from build123d import *

# Parameters (mm, degrees)
SKETCH_1_R               = 7.5
EXTRUDE_1_DEPTH          = 5
SKETCH_2_R               = 7.5
SKETCH_2_R_2             = 2
EXTRUDE_2_DEPTH          = 3
SKETCH_3_R               = 32.5
SKETCH_3_R_2             = 22.5
EXTRUDE_3_DEPTH          = 12
EXTRUDE_3_DEPTH_BACK     = 15
REVOLVE_1_ANGLE          = 12
PATTERN_CIRCULAR_1_COUNT = 10
SKETCH_5_R               = 4.5
CUT_EXTRUDE_1_DEPTH      = 2
FILLET_1_R               = 1


with BuildPart() as part:
    # Sketch 1 → Extrude 1 (new body)
    with BuildSketch(Plane.XY):
        Circle(SKETCH_1_R)
        Polygon((-6.92820323, 0), (-3.464101615, -6), (3.464101615, -6), (6.92820323, 0), (3.464101615, 6), (-3.464101615, 6), align=None, mode=Mode.SUBTRACT)
    extrude(amount=EXTRUDE_1_DEPTH)

    # Sketch 2 → Extrude 2 (add)
    with BuildSketch(Plane.XY):
        Circle(SKETCH_2_R)
        Circle(SKETCH_2_R_2, mode=Mode.SUBTRACT)
    extrude(amount=-EXTRUDE_2_DEPTH)



with BuildPart() as body_2:
    # Sketch 3 → Extrude 3 (new body, two sides)
    with BuildSketch(Plane.XY) as extrude_3_sk:
        Circle(SKETCH_3_R)
        Circle(SKETCH_3_R_2, mode=Mode.SUBTRACT)
    extrude(amount=EXTRUDE_3_DEPTH)
    extrude(extrude_3_sk.sketch, amount=-EXTRUDE_3_DEPTH_BACK)


with BuildPart() as part_1:
    add(part.part)

    add(body_2.part)  # Revolve 1 merges body 2
    # Sketch 4 → Revolve 1 (revolve)
    with BuildSketch(Plane(origin=(0, 0, 0), x_dir=(0, 0, -1), z_dir=(1, 0, 0))):
        with BuildLine():
            Line((-5, 7.5), (3, 7.5))
            ThreePointArc((3, 7.5), (7.415092079, 16.267926336), (15, 22.5))
            Line((15, 22.5), (7, 22.5))
            ThreePointArc((7, 22.5), (0.420622129, 15.463502297), (-5, 7.5))
        make_face()
    revolve_1 = revolve(axis=Axis((0, 0, -16.35), (0, 0, 1)), revolution_arc=REVOLVE_1_ANGLE)

    # Pattern Circular 1: Revolve 1 ×10 about axis
    pattern_circular_1_axis = Axis((0, 0, 0), (0, 0, 1))
    for i in range(1, PATTERN_CIRCULAR_1_COUNT):
        add(revolve_1.rotate(pattern_circular_1_axis, i * 360 / PATTERN_CIRCULAR_1_COUNT))

    # Sketch 5 → Cut-Extrude 1 (cut)
    with BuildSketch(Plane(origin=(0, 0, -3), x_dir=(-1, 0, 0), z_dir=(0, 0, -1))):
        Circle(SKETCH_5_R)
    extrude(amount=-CUT_EXTRUDE_1_DEPTH, mode=Mode.SUBTRACT)

    # Fillet 1
    fillet_1_edges = [part_1.edges().sort_by_distance(p)[0] for p in [
        (-32.5, 0, -15),
        (-32.5, 0, 12),
    ]]
    fillet(fillet_1_edges, radius=FILLET_1_R)


solid = part_1.part
Build history of the part. All positions in model axes, mm. A direction names the side the tool comes from. Coordinates: 2 decimals unless noted, no trailing zeros. Write item = value, one per line. Start each with the question number.
1) Two-plate mould, pull along X, no slides. Class faces 4 (the face through (-5.22, -2.96, 2.46)), 5 (the face through (31, 9.76, -1.32)): pulls with the +X half, pulls with the -X half, needs draft (parallel to the pull), parting line crosses it, or undercut.
2) Saw through at A-A on y = -13. Count the separate pieces of the cut face and the enclosed holes in it, then the cut area to 3 significant figures.
3) Wall check: line 1 along X through (y, z) = (9, -2); line 2 along X through (y, z) = (14, 4.5); line 3 along X through (y, z) = (1.5, -12.25). Give the ranges that are in metal, low to high. Write a range as from..to.
4) Flat gauge pins, fed straight in: pin 1 Ø12 at (x, z) = (19.5, -4) entering from -Y; pin 2 Ø12 at (y, z) = (-17, -3.5) entering from -X; pin 3 Ø10 at (x, y) = (-24.5, -23) entering from -Z; pin 4 Ø13 at (x, y) = (3.5, -1) entering from +Z. Where does each tip first touch, or does it go through?
5) 3-axis set-ups, long thin cutter, end or side, ignore diameter. For faces 1 (the face through (5.22, 2.96, 2.46)), 2 (the face through (-10.76, 9.69, -3.47)), 3 (the face through (-2, -1, -1)): which of +Z, -Z, +X, -X, +Y, -Y reach the whole face in a straight line?
From the geometry:
q1.face_4 = undercut
q1.face_5 = parting line crosses it
q2.separate_pieces = 5
q2.enclosed_holes = 0
q2.area = 690 mm^2
q3.line_1 = -31.23..-20.62, -10..-6.54, -1.91..0, 4.01..6.54, 20.62..31.23
q3.line_2 = -29.33..-17.61, 17.61..29.33
q3.line_3 = -32.47..-22.45, 22.45..32.47
q4.pin_1 = -29.56
q4.pin_2 = -30.58
q4.pin_3 = -15
q4.pin_4 = 5
q5.face_1 = +Z
q5.face_2 = +Z, -Z
q5.face_3 = -Z
